Work out the finished part from the listing and answer in its coordinate system (mm). Round coordinates to 2 decimals unless told otherwise and drop trailing zeros. Write each loop counter-clockwise with the first axis right and the second up, starting at its lowest first coordinate (ties: lowest second). Pieces come first, ordered by that corner, then holes.
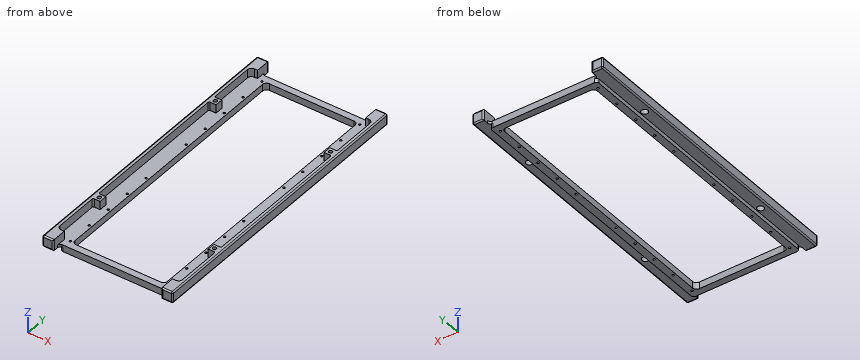
from build123d import *

# Parameters (mm, degrees)
SKETCH1_W             = 8.5
SKETCH1_H             = 8.5
BOSS_EXTRUDE1_DEPTH   = 227
SKETCH2_W             = 2
SKETCH2_H             = 214
BOSS_EXTRUDE2_DEPTH   = 50
BOSS_EXTRUDE3_DEPTH   = 3.18
CUT_EXTRUDE1_DEPTH    = 233.734660934
FILLET1_R             = 2
FILLET2_R             = 1
CUT_EXTRUDE2_DEPTH    = 6.5
M2X0_4_TAPPED_HOLE1_D = 1.6
SKETCH8_R             = 1.375
CUT_EXTRUDE3_DEPTH    = 233.596754062
SKETCH9_R             = 2.5
CUT_EXTRUDE4_DEPTH    = 4.75
LPATTERN1_COUNT       = 2
LPATTERN1_PITCH       = 88.5
LPATTERN1_COUNT_DIR2  = 2
LPATTERN1_PITCH_DIR2  = 122.4


with BuildPart() as part:
    # Sketch1 → Boss-Extrude1 (new body)
    with BuildSketch(Plane(origin=(0, 0, 0), x_dir=(1, 0, 0), z_dir=(0, 1, 0))):
        with Locations((45.75, 0)):
            Rectangle(SKETCH1_W, SKETCH1_H)
    boss_extrude1 = extrude(amount=BOSS_EXTRUDE1_DEPTH)

    # Sketch2 → Boss-Extrude2 (add)
    with BuildSketch(Plane.ZY.offset(-41.5)):
        with Locations((-3.25, 113.5)):
            Rectangle(SKETCH2_W, SKETCH2_H)
    boss_extrude2 = extrude(amount=BOSS_EXTRUDE2_DEPTH)

    # Mirror2: Boss-Extrude1, Boss-Extrude2 across plane
    add(boss_extrude1.mirror(Plane(origin=(0, 0, 0), x_dir=(0, 0, 1), z_dir=(1, 0, 0))))
    add(boss_extrude2.mirror(Plane(origin=(0, 0, 0), x_dir=(0, 0, 1), z_dir=(1, 0, 0))))

    # Sketch3 → Boss-Extrude3 (add)
    with BuildSketch(Plane(origin=(0, 0, -4.25), x_dir=(-1, 0, 0), z_dir=(0, 0, -1))):
        with BuildLine():
            Line((-39, 6.5), (39, 6.5))
            ThreePointArc((39, 6.5), (40.414213562, 7.085786438), (41, 8.5))
            Line((41, 8.5), (41, 218.5))
            ThreePointArc((41, 218.5), (40.414213562, 219.914213562), (39, 220.5))
            Line((39, 220.5), (-39, 220.5))
            ThreePointArc((-39, 220.5), (-40.414213562, 219.914213562), (-41, 218.5))
            Line((-41, 218.5), (-41, 8.5))
            ThreePointArc((-41, 8.5), (-40.414213562, 7.085786438), (-39, 6.5))
        make_face()
    extrude(amount=BOSS_EXTRUDE3_DEPTH)

    # Sketch4 → Cut-Extrude1 (cut, through all)
    with BuildSketch(Plane(origin=(0, 0, -7.43), x_dir=(-1, 0, 0), z_dir=(0, 0, -1))):
        with BuildLine():
            Line((-32.5, 11.5), (32.5, 11.5))
            ThreePointArc((32.5, 11.5), (34.621320344, 12.378679656), (35.5, 14.5))
            Line((35.5, 14.5), (35.5, 212.5))
            ThreePointArc((35.5, 212.5), (34.621320344, 214.621320344), (32.5, 215.5))
            Line((32.5, 215.5), (-32.5, 215.5))
            ThreePointArc((-32.5, 215.5), (-34.621320344, 214.621320344), (-35.5, 212.5))
            Line((-35.5, 212.5), (-35.5, 14.5))
            ThreePointArc((-35.5, 14.5), (-34.621320344, 12.378679656), (-32.5, 11.5))
        make_face()
    extrude(amount=-CUT_EXTRUDE1_DEPTH, mode=Mode.SUBTRACT)

    # Fillet1
    fillet1_edges = [part.edges().sort_by_distance(p)[0] for p in [
        (41.5, 6.5, -3.25),
        (-41.5, 6.5, -3.25),
        (41.5, 220.5, -3.25),
        (-41.5, 220.5, -3.25),
    ]]
    fillet(fillet1_edges, radius=FILLET1_R)

    # Fillet2
    fillet2_edges = [part.edges().sort_by_distance(p)[0] for p in [
        (41.5, 227, 0),
        (45.75, 227, 4.25),
        (-41.5, 227, 0),
        (-50, 227, 0),
        (-50, 113.5, -4.25),
        (-45.75, 227, -4.25),
        (-45.75, 227, 4.25),
        (-50, 113.5, 4.25),
        (-50, 0, 0),
        (-45.75, 0, -4.25),
        (-41.5, 0, 0),
        (-45.75, 0, 4.25),
        (50, 227, 0),
        (45.75, 0, 4.25),
        (41.5, 0, 0),
        (45.75, 0, -4.25),
        (50, 0, 0),
        (45.75, 227, -4.25),
        (50, 113.5, 4.25),
        (50, 113.5, -4.25),
    ]]
    fillet(fillet2_edges, radius=FILLET2_R)

    # Sketch5 → Cut-Extrude2 (cut)
    with BuildSketch(Plane.XY.offset(4.25)):
        with BuildLine():
            Line((-44, 11.5), (44, 11.5))
            ThreePointArc((44, 11.5), (46.121320344, 12.378679656), (47, 14.5))
            Line((47, 14.5), (47, 48.3))
            ThreePointArc((47, 48.3), (46.707106781, 49.007106781), (46, 49.3))
            Line((46, 49.3), (41.5, 49.3))
            Line((41.5, 49.3), (41.5, 55.3))
            Line((41.5, 55.3), (46, 55.3))
            ThreePointArc((46, 55.3), (46.707106781, 55.592893219), (47, 56.3))
            Line((47, 56.3), (47, 170.7))
            ThreePointArc((47, 170.7), (46.707106781, 171.407106781), (46, 171.7))
            Line((46, 171.7), (41.5, 171.7))
            Line((41.5, 171.7), (41.5, 177.7))
            Line((41.5, 177.7), (46, 177.7))
            ThreePointArc((46, 177.7), (46.707106781, 177.992893219), (47, 178.7))
            Line((47, 178.7), (47, 212.5))
            ThreePointArc((47, 212.5), (46.121320344, 214.621320344), (44, 215.5))
            Line((44, 215.5), (-44, 215.5))
            ThreePointArc((-44, 215.5), (-46.121320344, 214.621320344), (-47, 212.5))
            Line((-47, 212.5), (-47, 178.7))
            ThreePointArc((-47, 178.7), (-46.707106781, 177.992893219), (-46, 177.7))
            Line((-46, 177.7), (-41.5, 177.7))
            Line((-41.5, 177.7), (-41.5, 171.7))
            Line((-41.5, 171.7), (-46, 171.7))
            ThreePointArc((-46, 171.7), (-46.707106781, 171.407106781), (-47, 170.7))
            Line((-47, 170.7), (-47, 56.3))
            ThreePointArc((-47, 56.3), (-46.707106781, 55.592893219), (-46, 55.3))
            Line((-46, 55.3), (-41.5, 55.3))
            Line((-41.5, 55.3), (-41.5, 49.3))
            Line((-41.5, 49.3), (-46, 49.3))
            ThreePointArc((-46, 49.3), (-46.707106781, 49.007106781), (-47, 48.3))
            Line((-47, 48.3), (-47, 14.5))
            ThreePointArc((-47, 14.5), (-46.121320344, 12.378679656), (-44, 11.5))
        make_face()
    extrude(amount=-CUT_EXTRUDE2_DEPTH, mode=Mode.SUBTRACT)

    # M2x0.4 Tapped Hole1 (through all)
    with Locations(Plane(origin=(0, 0, -7.43), x_dir=(-1, 0, 0), z_dir=(0, 0, -1))):
        with Locations((-37.5, 214.7), (37.5, 214.7), (37.5, 194.7), (37.5, 174.7), (37.5, 154.7), (37.5, 134.7), (-37.5, 194.7), (-37.5, 174.7), (-37.5, 154.7), (-37.5, 134.7), (-37.5, 12.3), (-37.5, 32.3), (-37.5, 52.3), (-37.5, 72.3), (-37.5, 92.3), (37.5, 92.3), (37.5, 72.3), (37.5, 52.3), (37.5, 32.3), (37.5, 12.3)):
            Hole(M2X0_4_TAPPED_HOLE1_D / 2)

    # Sketch8 → Cut-Extrude3 (cut, through all)
    with BuildSketch(Plane(origin=(0, 0, -4.25), x_dir=(-1, 0, 0), z_dir=(0, 0, -1))):
        with Locations((-44.25, 174.7)):
            Circle(SKETCH8_R)
    cut_extrude3 = extrude(amount=-CUT_EXTRUDE3_DEPTH, mode=Mode.SUBTRACT)

    # Sketch9 → Cut-Extrude4 (cut)
    with BuildSketch(Plane(origin=(0, 0, -4.25), x_dir=(-1, 0, 0), z_dir=(0, 0, -1))):
        with Locations((-44.25, 174.7)):
            Circle(SKETCH9_R)
    cut_extrude4 = extrude(amount=-CUT_EXTRUDE4_DEPTH, mode=Mode.SUBTRACT)

    # LPattern1: Cut-Extrude3, Cut-Extrude4 2 × 2
    with Locations(*[(-i * LPATTERN1_PITCH, -j * LPATTERN1_PITCH_DIR2, 0) for i in range(LPATTERN1_COUNT) for j in range(LPATTERN1_COUNT_DIR2) if (i, j) != (0, 0)]):
        add(cut_extrude3, mode=Mode.SUBTRACT)
        add(cut_extrude4, mode=Mode.SUBTRACT)


solid = part.part
Q1. Find section B-B (x = -10). Determine the outline of the cut face in (y, z).
Q2. Find section A-A (y = 41.5). Determine the outline of the cut face in (x, z), plus the area to 3 significant figures.
Q3. Find the intervals of material crossed by L1, parallel to X at y = 92.3, z = -5.1; L2, parallel to X at y = 52.3, z = -0.9; L3, parallel to X at y = 187, z = 1.25, in increasing order.
Q4. Given pin 1 (2.5 mm diameter, centred on x = 37.5, y = 52.3, fed in from +Z); pin 2 (1 mm diameter, centred on x = 18.5, z = -4, fed in from -Y); pin 3 (1 mm diameter, centred on y = 201.5, z = -6, fed in from -X), each flat-ended and moving along its own axis, determine where each tip first touches the part or whether it passes through.
Report:
1. outline: (6.5, -7.43) - (11.5, -7.43) - (11.5, -2.25) - (6.5, -2.25) - close; (215.5, -7.43) - (220.5, -7.43) - (220.5, -2.25) - (215.5, -2.25) - close
2. outline: (-50, -3.25) arc R1 ccw to (-49, -4.25) - (-41, -4.25) - (-41, -7.43) - (-35.5, -7.43) - (-35.5, -2.25) - (-47, -2.25) - (-47, 4.25) - (-49, 4.25) arc R1 ccw to (-50, 3.25) - close; (35.5, -7.43) - (41, -7.43) - (41, -4.25) - (49, -4.25) arc R1 ccw to (50, -3.25) - (50, 3.25) arc R1 ccw to (49, 4.25) - (47, 4.25) - (47, -2.25) - (35.5, -2.25) - close
2. area: 131 mm2
3. L1: x = -41 to -38.3, -36.7 to -35.5, 35.5 to 36.7, 38.3 to 41
3. L2: x = -50 to -46.75, -41.75 to -41.5, 41.5 to 41.75, 46.75 to 50
3. L3: x = -50 to -47, 47 to 50
4. pin 1: stops at z = -2.25
4. pin 2: stops at y = 6.5
4. pin 3: stops at x = -41
